Can you work these out from the model? Positions are in its coordinate system, mm. Round coordinates to 2 decimals unless told otherwise and drop trailing zeros. Write each loop counter-clockwise with the first axis right and the second up, starting at its lowest first coordinate (ties: lowest second). Pieces come first, ordered by that corner, then holes. Notation, with made-up numbers: M -25,72.5 L 6,72.5 A23 cw 6,104.5 Z; hole C 46.5,26 d10. An arc over 180 degrees is marked long. Answer as a JSON object with one key per item and string values. Group by question number.
1) I'm going to push flat-ended pins straight in: pin 1 Ø10 at (x, z) = (10, 23) entering from +Y; pin 2 Ø8 at (x, y) = (12.5, 6.5) entering from +Z; pin 3 Ø9.5 at (y, z) = (-0.5, 183.5) entering from -X; pin 4 Ø6 at (y, z) = (11.5, -121.5) entering from +X. Where does each tip first touch, or does it pass through?
2) Suppose I cut it at A-A, the plane z = -135.5. Write out the boundary of the cut face in (x, y).
3) Please list where these lines run through material, in increasing order: L1, parallel to X at y = 3.5, z = -31; L2, parallel to Z at x = 3.5, y = 13. Write a range as [from, to].
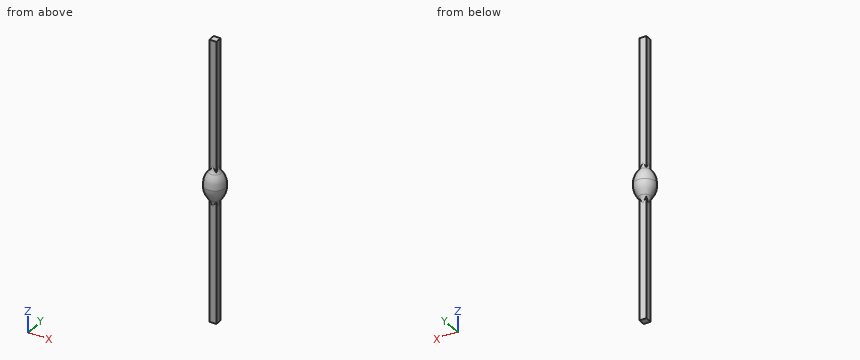
from build123d import *

# Parameters (mm, degrees)
F3_DEPTH      = 210
F3_DEPTH_BACK = 25
F5_DEPTH      = 194
F5_DEPTH_BACK = 25


with BuildPart() as f1:
    # F0 (on Front) → F1 (revolve)
    with BuildSketch(Plane.XZ):
        with BuildLine():
            Line((6, 40), (0, 40))
            Line((0, 40), (0, -40))
            Line((0, -40), (6, -40))
            Line((6, -40), (6, -35))
            ThreePointArc((6, -35), (7.121945325, -28.3955279025), (10.3619051686, -22.5320414644))
            ThreePointArc((10.3619051686, -22.5320414644), (16.1478700246, -11.9337677658), (17.9879737223, 0))
            ThreePointArc((17.9879737223, 0), (16.1478700246, 11.9337677658), (10.3619051686, 22.5320414644))
            ThreePointArc((10.3619051686, 22.5320414644), (7.121945325, 28.3955279025), (6, 35))
            Line((6, 35), (6, 40))
        make_face()
    revolve(axis=Axis((0, 0, 0), (0, 0, -1)))

    # F2 (on face) → F3 (join, two sides)
    with BuildSketch(Plane.XY.offset(40)) as f3_sk:
        with BuildLine():
            Line((6, 0), (6, 6))
            Line((6, 6), (0, 6))
            ThreePointArc((0, 6), (4.2426406871, 4.2426406871), (6, 0))
        make_face()
        with BuildLine():
            ThreePointArc((-6, 0), (-4.2426406871, 4.2426406871), (0, 6))
            Line((0, 6), (-6, 6))
            Line((-6, 6), (-6, 0))
        make_face()
        with BuildLine():
            ThreePointArc((0, -6), (-4.2426406871, -4.2426406871), (-6, 0))
            Line((-6, 0), (-6, -6))
            Line((-6, -6), (0, -6))
        make_face()
        with BuildLine():
            Line((6, -6), (6, 0))
            ThreePointArc((6, 0), (4.2426406871, -4.2426406871), (0, -6))
            Line((0, -6), (6, -6))
        make_face()
        with BuildLine():
            ThreePointArc((6, 0), (4.2426406871, 4.2426406871), (0, 6))
            ThreePointArc((0, 6), (-4.2426406871, 4.2426406871), (-6, 0))
            ThreePointArc((-6, 0), (-4.2426406871, -4.2426406871), (0, -6))
            ThreePointArc((0, -6), (4.2426406871, -4.2426406871), (6, 0))
        make_face()
    extrude(amount=F3_DEPTH)
    extrude(f3_sk.sketch, amount=-F3_DEPTH_BACK)

    # F4 (on face) → F5 (join, two sides)
    with BuildSketch(Plane(origin=(0, 0, -40), x_dir=(1, 0, 0), z_dir=(0, 0, -1))) as f5_sk:
        with BuildLine():
            Line((6, 0), (6, 6))
            Line((6, 6), (0, 6))
            ThreePointArc((0, 6), (4.2426406871, 4.2426406871), (6, 0))
        make_face()
        with BuildLine():
            ThreePointArc((-6, 0), (-4.2426406871, 4.2426406871), (0, 6))
            Line((0, 6), (-6, 6))
            Line((-6, 6), (-6, 0))
        make_face()
        with BuildLine():
            ThreePointArc((6, 0), (4.2426406871, 4.2426406871), (0, 6))
            ThreePointArc((0, 6), (-4.2426406871, 4.2426406871), (-6, 0))
            ThreePointArc((-6, 0), (-4.2426406871, -4.2426406871), (0, -6))
            ThreePointArc((0, -6), (4.2426406871, -4.2426406871), (6, 0))
        make_face()
        with BuildLine():
            Line((6, -6), (6, 0))
            ThreePointArc((6, 0), (4.2426406871, -4.2426406871), (0, -6))
            Line((0, -6), (6, -6))
        make_face()
        with BuildLine():
            ThreePointArc((0, -6), (-4.2426406871, -4.2426406871), (-6, 0))
            Line((-6, 0), (-6, -6))
            Line((-6, -6), (0, -6))
        make_face()
    extrude(amount=F5_DEPTH)
    extrude(f5_sk.sketch, amount=-F5_DEPTH_BACK)


solid = f1.part
Results:
{
 "1": {"pin 1": "y = 10.77", "pin 2": "z = 22.88", "pin 3": "x = -6", "pin 4": "through"},
 "2": {"outline": "M -6,-6 L 6,-6 L 6,6 L -6,6 Z"},
 "3": {"L1": "[-6, 6]", "L2": "[-17.94, 17.94]"}
}
